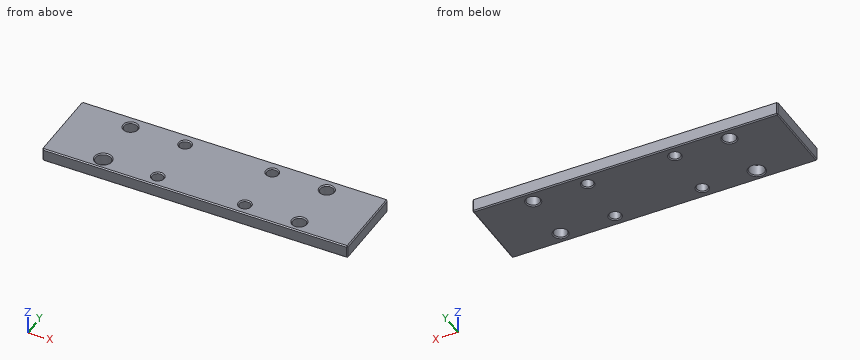
Autodesk Fusion 360 part; units mm, degrees
sketch "Top" plane through (0, 0, 0) normal (0, 0, 1) x (1, 0, 0)
  line L0 (-70, 0) -> (70, 0)
  line L1 (70, 0) -> (70, 35)
  line L2 (70, 35) -> (-70, 35)
  line L3 (-70, 35) -> (-70, 0)
  line L4 (-45, 29.5) -> (45, 29.5) construction
  line L5 (45, 29.5) -> (45, 5.5) construction
  line L6 (45, 5.5) -> (-45, 5.5) construction
  line L7 (-45, 5.5) -> (-45, 29.5) construction
  line L8 (70, 24.75) -> (45, 24.75) construction
  line L9 (-70, 24.75) -> (-45, 24.75) construction
  line L10 (20, 35) -> (20, 29.5) construction
  line L11 (9.991, 5.5) -> (9.991, 0) construction
  line L12 (-20, 29.5) -> (20, 29.5) construction
  line L13 (20, 29.5) -> (20, 5.5) construction
  line L14 (20, 5.5) -> (-20, 5.5) construction
  line L15 (-20, 5.5) -> (-20, 29.5) construction
  line L16 (20, 14.3708) -> (45, 14.3708) construction
  line L17 (-20, 14.3708) -> (-45, 14.3708) construction
  circle A0 centre (-45, 29.5) radius 3
  circle A1 centre (-45, 5.5) radius 3.5
  circle A2 centre (45, 29.5) radius 3
  circle A3 centre (45, 5.5) radius 3
  circle A4 centre (20, 29.5) radius 2.5
  circle A5 centre (-20, 29.5) radius 2.5
  circle A6 centre (20, 5.5) radius 2.5
  circle A7 centre (-20, 5.5) radius 2.5
  dimension "d1" = 140
  dimension "d2" = 35
  dimension "d3" = 70
  dimension "d4" = 90
  dimension "d5" = 24
  dimension "d6" = 40
  dimension "d7" = 6
  dimension "d8" = 7
  dimension "d9" = 6
  dimension "d10" = 6
  dimension "d11" = 5
  dimension "d13" = 5
  dimension "d15" = 35
  dimension "d16" = 40
  dimension "d18" = 24
  dimension "d19" = 5
  dimension "d20" = 5
extrude "Extrude1" add sketch "Top" along normal blind 6
chamfer "Chamfer1" distance 0.5 angle 45 15 edges at (0, 35, 0) (-70, 17.5, 0) (0, 0, 0) (70, 17.5, 0) (70, 35, 3) (-70, 35, 3) (-70, 0, 3) (-47.797, 30.5848, 0) (-48.2631, 6.7657, 0) (-22.3308, 6.404, 0) (-22.3308, 30.404, 0) (17.6692, 30.404, 0) (17.6692, 6.404, 0) (42.203, 6.5848, 0) (42.203, 30.5848, 0)
chamfer "Chamfer2" distance 0.5 angle 45 11 edges at (0.25, 0, 6) (70, 0, 3.25) (70, 17.25, 6) (42.203, 30.5848, 6) (42.203, 6.5848, 6) (17.6692, 6.404, 6) (17.6692, 30.404, 6) (-22.3308, 30.404, 6) (-22.3308, 6.404, 6) (-48.2631, 6.7657, 6) (-47.797, 30.5848, 6)
For this review, take the finished solid that the model builds, in its own axes (mm). Round coordinates to 2 decimals unless told otherwise and drop trailing zeros. Write each loop counter-clockwise with the first axis right and the second up, starting at its lowest first coordinate (ties: lowest second). Pieces come first, ordered by that corner, then holes. Notation, with made-up numbers: (6, -11) - (27, -11) arc R18 ccw to (27, -5) - close; hole circle Ø10 at (-32, 43). An arc over 180 degrees is marked (long way). Write each question's results on one line, items separated by ' | '.
Item 1: Take a section at A-A on x = -20. State the section outline as (y, z) points, then the cut area to 3 significant figures.
Calculated:
outline: (0, 0.5) - (0.5, 0) - (2.5, 0) - (3, 0.5) - (3, 5.5) - (2.5, 6) - (0.5, 6) - (0, 5.5) - close; (8, 0.5) - (8.5, 0) - (26.5, 0) - (27, 0.5) - (27, 5.5) - (26.5, 6) - (8.5, 6) - (8, 5.5) - close; (32, 0.5) - (32.5, 0) - (34.5, 0) - (35, 0.5) - (35, 6) - (32.5, 6) - (32, 5.5) - close | area: 149 mm^2
Item 2: Take a section at C-C on x = -45. State the section outline as (y, z) points.
Calculated:
outline: (0, 0.5) - (0.5, 0) - (1.5, 0) - (2, 0.5) - (2, 5.5) - (1.5, 6) - (0.5, 6) - (0, 5.5) - close; (9, 0.5) - (9.5, 0) - (26, 0) - (26.5, 0.5) - (26.5, 5.5) - (26, 6) - (9.5, 6) - (9, 5.5) - close; (32.5, 0.5) - (33, 0) - (34.5, 0) - (35, 0.5) - (35, 6) - (33, 6) - (32.5, 5.5) - close
Item 3: Take a section at B-B on z = 2.75. Count the separate pieces of the cut face and the enclosed holes in it, then the cut area to 3 significant figures.
Calculated:
separate pieces: 1 | enclosed holes: 8 | area: 4,700 mm^2
Item 4: To check wall thickness, follow line 1 along Y through (x, z) = (-20, 4.5); line 2 along Y through (x, z) = (45, 2.4); line 3 along X through (y, z) = (5, 3). State the ranges of each line that lie inside material, in increasing order. Write a range as from..to.
Calculated:
line 1: y = 0..3, 8..27, 32..35 | line 2: y = 0..2.5, 8.5..26.5, 32.5..35 | line 3: x = -70..-48.46, -41.54..-22.45, -17.55..17.55, 22.45..42.04, 47.96..70
